from build123d import *

# Parameters (mm, degrees)
SKETCH1_W           = 41.275
SKETCH1_H           = 1.7272
SKETCH1_W_2         = 39.37
SKETCH1_H_2         = 7.1628
BOSS_EXTRUDE1_DEPTH = 1.7272


with BuildPart() as part:
    # Sketch1 → Boss-Extrude1 (new body)
    with BuildSketch(Plane.XY):
        Polygon((-112.395, -12.7), (-114.3, -12.7), (-114.3, -11.8872), (-116.0272, -11.8872), (-116.0272, -9.8552), (-114.3, -9.8552), (-114.3, 8.4328), (-116.0272, 8.4328), (-116.0272, 10.4648), (-114.3, 10.4648), (-114.3, 12.7), (114.3, 12.7), (114.3, 10.4648), (116.0272, 10.4648), (116.0272, 8.4328), (114.3, 8.4328), (114.3, -9.8552), (116.0272, -9.8552), (116.0272, -11.8872), (114.3, -11.8872), (114.3, -12.7), (112.395, -12.7), (112.395, -10.9728), (71.12, -10.9728), (71.12, -12.7), (-71.12, -12.7), (-71.12, -10.9728), (-112.395, -10.9728), align=None)
        Polygon((67.31, -6.201073431), (11.500339125, 0), (67.31, 6.201073431), align=None, mode=Mode.SUBTRACT)
        Polygon((-67.31, 8.89), (-1.27, 8.89), (-1.27, 1.418926569), (-67.31, 8.756704347), align=None, mode=Mode.SUBTRACT)
        Polygon((-67.31, -8.89), (-1.27, -8.89), (-1.27, -1.418926569), (-67.31, -8.756704347), align=None, mode=Mode.SUBTRACT)
        Polygon((67.31, 8.89), (67.31, 8.756704347), (1.27, 1.418926569), (1.27, 8.89), align=None, mode=Mode.SUBTRACT)
        Polygon((67.31, -8.756704347), (1.27, -1.418926569), (1.27, -8.89), (67.31, -8.89), align=None, mode=Mode.SUBTRACT)
        Polygon((-67.31, 6.201073431), (-67.31, -6.201073431), (-11.500339125, 0), align=None, mode=Mode.SUBTRACT)
        with Locations((-91.7575, 5.9436)):
            Rectangle(SKETCH1_W, SKETCH1_H, mode=Mode.SUBTRACT)
        with Locations((91.7575, 5.9436)):
            Rectangle(SKETCH1_W, SKETCH1_H, mode=Mode.SUBTRACT)
        with Locations((90.805, -2.3114)):
            Rectangle(SKETCH1_W_2, SKETCH1_H_2, mode=Mode.SUBTRACT)
        with Locations((-90.805, -2.3114)):
            Rectangle(SKETCH1_W_2, SKETCH1_H_2, mode=Mode.SUBTRACT)
    extrude(amount=BOSS_EXTRUDE1_DEPTH)


solid = part.part
Input: part model. Units: mm. Frame: model coordinates. A direction names the side the tool comes from. Coordinates: 2 decimals unless noted, no trailing zeros. Loops run counter-clockwise (first coordinate to the right, second up) from the corner with the lowest first, then second, coordinate; pieces in that order, holes last.
(1) Section A-A on x = -96. Return the cut outline in (y, z), then the cut area to 3 significant figures.
(2) Section C-C on z = 1.25. Count the separate pieces of the cut face and the enclosed holes in it, then the cut area to 3 significant figures.
(3) Section B-B on x = -58. Return the cut outline in (y, z), then the cut area to 3 significant figures.
(4) Pull-direction query (X, two-part tool) for faces 1 (the face through (-39.015, 3.057, 0.852)), 2 (the face through (-33.828, -5.036, 0.852)), 3 (the face through (2, 0, 0)); classes: released by +X, released by -X, zero draft, split by the parting line, or undercut.
(5) Material intervals for probe 1 along Y at (x, z) = (71.5, 0.65); probe 2 along Y at (x, z) = (-7, 1); probe 3 along Y at (x, z) = (39.5, 1.25), sorted ascending.
(6) First-contact query: pin 1 Ø0.5 at (y, z) = (1, 1) entering from +X; pin 2 Ø0.9 at (y, z) = (-2, 1) entering from -X. Flat tips, straight axial feed; report the tip coordinate or a pass-through.
(7) Set-up query: faces 4 (the face through (2, 0, 1.727)), 5 (the face through (34.75, 5.14, 0.85)). Return all of +Z, -Z, +X, -X, +Y, -Y with unobstructed straight access to the full face (end or side cutting, diameter ignored); none if empty.
Data:
1. outline: (-10.97, 0) - (-5.89, 0) - (-5.89, 1.73) - (-10.97, 1.73) - close; (1.27, 0) - (5.08, 0) - (5.08, 1.73) - (1.27, 1.73) - close; (6.81, 0) - (12.7, 0) - (12.7, 1.73) - (6.81, 1.73) - close
1. area: 25.5 mm2
2. separate pieces: 1
2. enclosed holes: 10
2. area: 3,270 mm2
3. outline: (-12.7, 0) - (-8.89, 0) - (-8.89, 1.73) - (-12.7, 1.73) - close; (-7.72, 0) - (-5.17, 0) - (-5.17, 1.73) - (-7.72, 1.73) - close; (5.17, 0) - (7.72, 0) - (7.72, 1.73) - (5.17, 1.73) - close; (8.89, 0) - (12.7, 0) - (12.7, 1.73) - (8.89, 1.73) - close
3. area: 22.0 mm2
4. face 1: undercut
4. face 2: undercut
4. face 3: zero draft
5. probe 1: y = -10.97 to -5.89, 1.27 to 5.08, 6.81 to 12.7
5. probe 2: y = -12.7 to -8.89, -2.06 to 2.06, 8.89 to 12.7
5. probe 3: y = -12.7 to -8.89, -5.67 to -3.11, 3.11 to 5.67, 8.89 to 12.7
6. pin 1: stops at x = 114.3
6. pin 2: stops at x = -114.3
7. face 4: +Z, +X, -X, +Y, -Y
7. face 5: +Z, -Z
